Design review of the part shown in the three views and the two pictorial views. Dimensions are in mm from the part's minimum x, y and z. A direction names the side the tool comes from. Give positions to 0.01 mm unless a question says otherwise; leave off trailing zeros. Write each loop counter-clockwise with the first axis right and the second up, starting at its lowest first coordinate (ties: lowest second). Pieces come first, ordered by that corner, then holes.
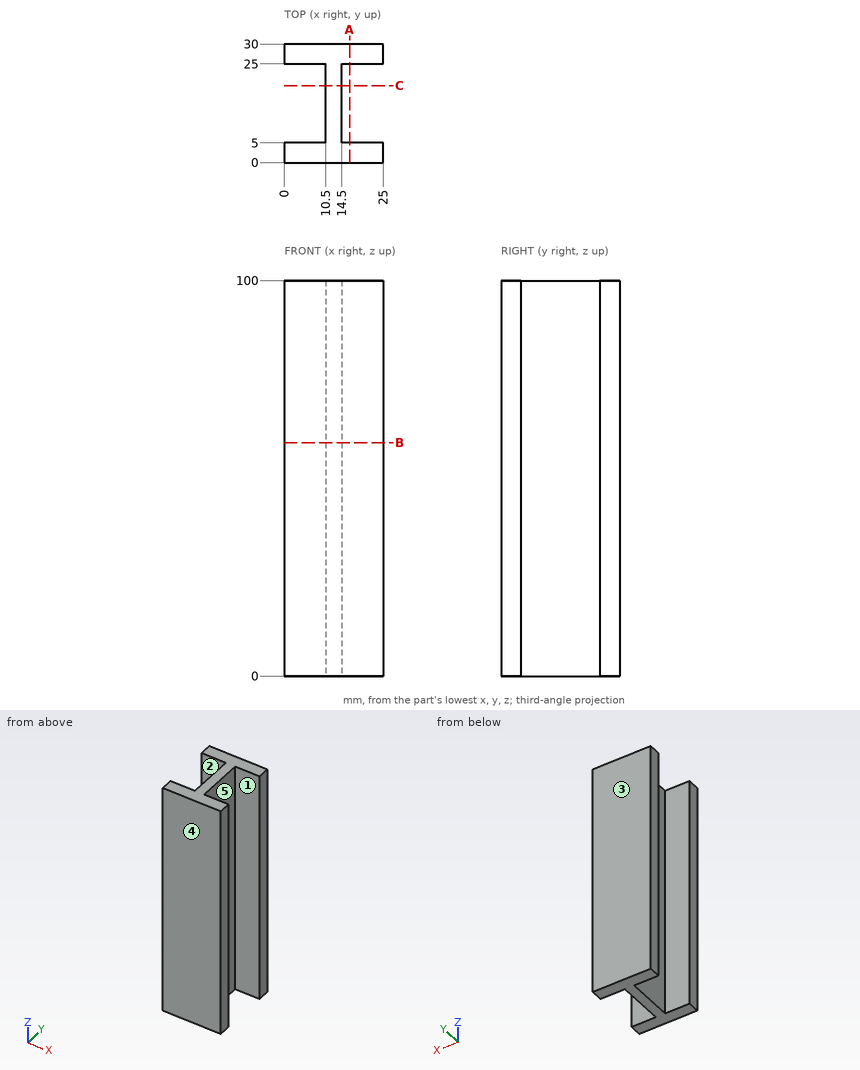
(1) Consider section A-A, the plane x = 16.5. Give the boundary of the cut face in (y, z).
Resolved:
outline: (0, 0) - (5, 0) - (5, 100) - (0, 100) - close; (25, 0) - (30, 0) - (30, 100) - (25, 100) - close
(2) Mouldability with a two-part tool opening along Y and no side actions: class the marked faces 3, 4 and 5 as pulls with the +Y half, pulls with the -Y half, needs draft (parallel to the pull), parting line crosses it, or undercut.
Resolved:
face 3: pulls with the +Y half
face 4: pulls with the -Y half
face 5: undercut
(3) Consider section B-B, the plane z = 59. Give the boundary of the cut face in (x, y).
Resolved:
outline: (0, 0) - (25, 0) - (25, 5) - (14.5, 5) - (14.5, 25) - (25, 25) - (25, 30) - (0, 30) - (0, 25) - (10.5, 25) - (10.5, 5) - (0, 5) - close
(4) Tool access review of the marked faces 1 and 2: name each direction out of +Z, -Z, +X, -X, +Y, -Y from which nothing blocks a thin tool from reaching the whole face with its end or side.
Resolved:
face 1: +Z, -Z, +X
face 2: +Z, -Z, -X
(5) Consider section C-C, the plane y = 19.5. Give the boundary of the cut face in (x, z), then the cut area to 3 significant figures.
Resolved:
outline: (10.5, 0) - (14.5, 0) - (14.5, 100) - (10.5, 100) - close
area: 400 mm2
(6) To check wall thickness, follow L1, parallel to Y at x = 23.5, z = 15.5; L2, parallel to X at y = 7, z = 33. State the ranges of each line that lie inside material, in increasing order.
Resolved:
L1: y = 0 to 5, 25 to 30
L2: x = 10.5 to 14.5
(7) Clearance check with flat-ended pins moving along their axes: P1, Ø1.5, axis at y = 15.5, z = 74, coming from the +X side; P2, Ø3, axis at x = 7.5, y = 14.5, coming from the -Z side; P3, Ø10, axis at y = 14.5, z = 31, coming from the -X side. State where each tip first meets the part, or that it passes through.
Resolved:
P1: stops at x = 14.5
P2: passes through
P3: stops at x = 10.5
